Source: CAD feature listing. Evaluate the final solid. Frame: model axes, mm. A direction names the side the tool comes from. Coordinates: 2 decimals unless noted, no trailing zeros. Order: outer loops, then holes, each group sorted by start corner. A loop starts at its lowest first (then second) coordinate and runs counter-clockwise, first axis right, second up. Notation, with made-up numbers: (51, -31.75) - (60, -31.75) arc R21 cw to (60, -0.75) - close; hole circle Ø5 at (53, 54.5). An arc over 180 degrees is marked (long way). One line per question, with ' | ' between items. Start each with the question number.
(1) Access query for faces 1 (the flat face through (3, -5, 0.5)), 2 (the flat face through (17.9, -5.07, 5.06)). Directions: +Z, -Z, +X, -X, +Y, -Y. A direction counts if a zero-diameter tool reaches every point of the face in a straight line with its end or side. Return the directions, or none.
(2) Section B-B (z = 8.5). Return the cut outline in (x, y), then the cut area to 3 significant figures.
(3) Line query: line 1 along Z through (x, y) = (2, -0.75); line 2 along X through (y, z) = (-7, 5.75); line 3 along X through (y, z) = (-0.25, 1). Output: solid intervals per line, ascending.
(4) Section D-D (y = -5.25). Count the separate pieces of the cut face and the enclosed holes in it, then the cut area to 3 significant figures.
(5) Section C-C (x = 8.5). Return the cut outline in (y, z), then the cut area to 3 significant figures.
(6) Contact query for flat-ended pins moving along their axis: P1, Ø4, axis at x = 8, y = -3.5, coming from the -Z side; P2, Ø0.6, axis at y = -4, z = 0, coming from the +X side; P3, Ø4, axis at x = 4.5, y = -4, coming from the +Z side. Output: stop coordinate, or through.
(7) Section A-A (y = -1). Return the cut outline in (x, z).
from build123d import *

# Parameters (mm, degrees)
SKETCH2_W                                         = 10
SKETCH2_H                                         = 10
BOSS_EXTRUDE1_DEPTH                               = 0.5
BOSS_EXTRUDE2_DEPTH                               = 10
CSK_FOR_1_FLAT_HEAD_SOCKET_CAP_SCREW1_D           = 2.0574
CSK_FOR_1_FLAT_HEAD_SOCKET_CAP_SCREW1_CSINK_D     = 4.2672
CSK_FOR_1_FLAT_HEAD_SOCKET_CAP_SCREW1_CSINK_ANGLE = 82
CSK_FOR_1_FLAT_HEAD_SOCKET_CAP_SCREW2_D           = 2.0574
CSK_FOR_1_FLAT_HEAD_SOCKET_CAP_SCREW2_CSINK_D     = 4.2672
CSK_FOR_1_FLAT_HEAD_SOCKET_CAP_SCREW2_CSINK_ANGLE = 82


with BuildPart() as part:
    # Sketch2 → Boss-Extrude1 (new body)
    with BuildSketch(Plane.XY):
        with Locations((5, -5)):
            Rectangle(SKETCH2_W, SKETCH2_H)
    extrude(amount=BOSS_EXTRUDE1_DEPTH)

    # Sketch3 → Boss-Extrude2 (add)
    with BuildSketch(Plane.XZ.offset(10)):
        Polygon((8, 0.5), (23.588457268, 9.5), (25.588457268, 9.5), (10, 0.5), align=None)
    extrude(amount=-BOSS_EXTRUDE2_DEPTH)

    # CSK for #1 Flat Head Socket Cap Screw1 (through all)
    with Locations(Plane(origin=(0, 0, 0), x_dir=(-1, 0, 0), z_dir=(0, 0, -1))):
        with Locations((-5.362516401, -4.921292394)):
            CounterSinkHole(CSK_FOR_1_FLAT_HEAD_SOCKET_CAP_SCREW1_D / 2, CSK_FOR_1_FLAT_HEAD_SOCKET_CAP_SCREW1_CSINK_D / 2, counter_sink_angle=CSK_FOR_1_FLAT_HEAD_SOCKET_CAP_SCREW1_CSINK_ANGLE)

    # CSK for #1 Flat Head Socket Cap Screw2 (through all)
    with Locations(Plane(origin=(2.283493649, 0, -3.955127019), x_dir=(-0.866025404, 0, -0.5), z_dir=(0.5, 0, -0.866025404))):
        with Locations((-14.39146791, -4.879407471)):
            CounterSinkHole(CSK_FOR_1_FLAT_HEAD_SOCKET_CAP_SCREW2_D / 2, CSK_FOR_1_FLAT_HEAD_SOCKET_CAP_SCREW2_CSINK_D / 2, counter_sink_angle=CSK_FOR_1_FLAT_HEAD_SOCKET_CAP_SCREW2_CSINK_ANGLE)


solid = part.part
Response values:
1) face 1: +Z, -X, +Y, -Y | face 2: -Z, +X, +Y, -Y
2) outline: (21.86, -10) - (23.86, -10) - (23.86, 0) - (21.86, 0) - close | area: 20.0 mm²
3) line 1: z = 0 to 0.5 | line 2: x = 17.09 to 19.09 | line 3: x = 8.87 to 10.87
4) separate pieces: 3 | enclosed holes: 0 | area: 17.8 mm²
5) outline: (-10, 0) - (0, 0) - (0, 0.79) - (-10, 0.79) - close | area: 7.89 mm²
6) P1: stops at z = 0 | P2: stops at x = 10 | P3: stops at z = 0.5
7) outline: (0, 0) - (10, 0) - (10, 0.5) - (25.59, 9.5) - (23.59, 9.5) - (8, 0.5) - (0, 0.5) - close
